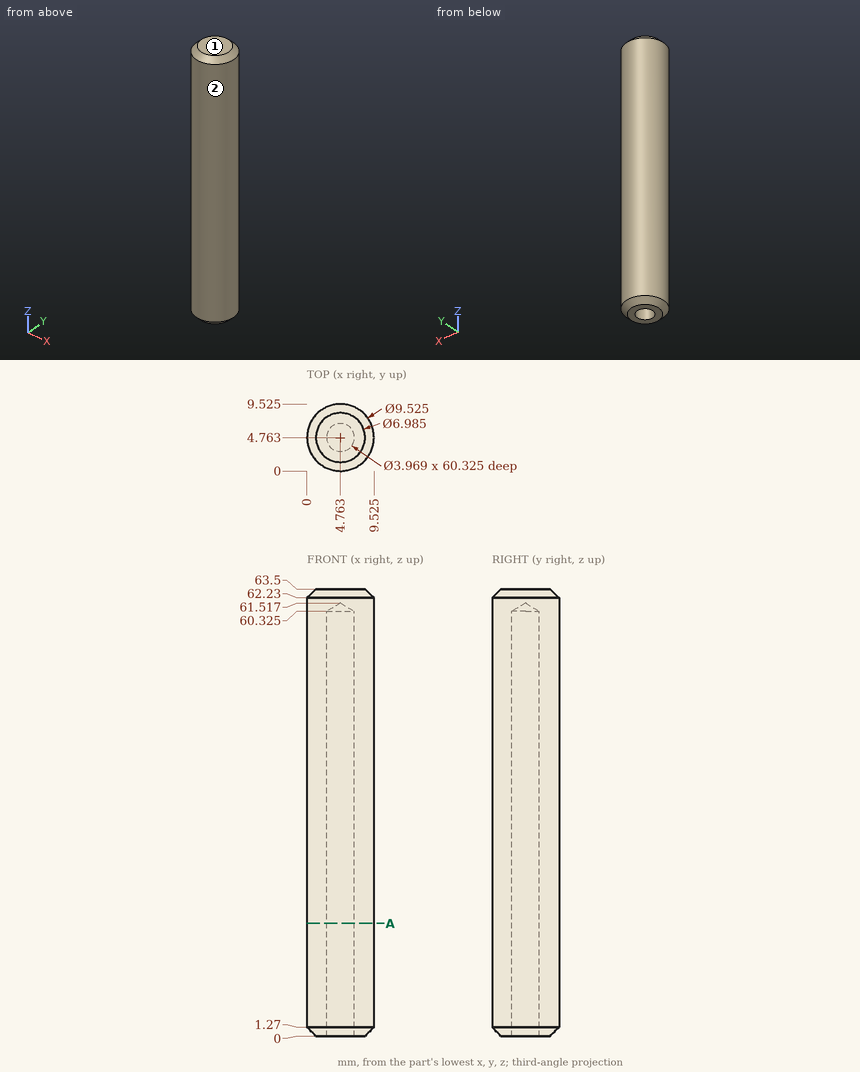
Drawing for the job (mm, zero at the part's lowest x, y, z). Round coordinates to 2 decimals unless told otherwise and drop trailing zeros. Loops run counter-clockwise (first coordinate to the right, second up) from the corner with the lowest first, then second, coordinate; pieces in that order, holes last. Notation, with made-up numbers: (-27, 2) - (-22, 2) arc R20 ccw to (-22, 15) - close; hole circle Ø1 at (23.5, 74.25). An arc over 180 degrees is marked (long way). Write each question's results on one line, items separated by ' | '.
(1) Mould opens along Y. For the marked faces 1 and 2 say: released by +Y, released by -Y, zero draft, split by the parting line, or undercut.
Answer below:
face 1: zero draft | face 2: split by the parting line
(2) Pin check, flat tips, straight feed: pin 1 (2 mm diameter, centred on y = 7.5, z = 50.5, fed in from +X); pin 2 (5 mm diameter, centred on y = 7, z = 20, fed in from +X) (1 decimal); pin 3 (1.5 mm diameter, centred on x = 7.5, z = 52.5, fed in from +Y). Stop position of each tip, or through.
Answer below:
pin 1: stops at x = 9.2 | pin 2: stops at x = 9.5 | pin 3: stops at y = 9.09
(3) Wall check: L1, parallel to Y at x = 4.75, z = 51.5 (1 decimal); L2, parallel to X at y = 6.5, z = 49.5 (1 decimal). Give the ranges that are in metal, low to high.
Answer below:
L1: y = 0 to 2.8, 6.7 to 9.5 | L2: x = 0.3 to 3.8, 5.7 to 9.2
(4) Saw through at A-A, the plane z = 16. List the corners of the cut face in (x, y) (1 decimal).
Answer below:
outline: circle Ø9.5 at (4.8, 4.8); hole circle Ø4 at (4.8, 4.8)
